Autodesk Inventor part; units mm, degrees
ref_plane "YZ Plane" through (0, 0, 0) normal (1, 0, 0) x (0, 1, 0)
ref_plane "XZ Plane" through (0, 0, 0) normal (0, 1, 0) x (-1, 0, 0)
ref_plane "XY Plane" through (0, 0, 0) normal (0, 0, 1) x (1, 0, 0)
sketch "Sketch2" plane through (0, 0, 0) normal (0, 0, 1) x (1, 0, 0)
  line L0 (0, 0) -> (19, 0)
  line L1 (19, 0) -> (19, 137)
  line L2 (19, 137) -> (0, 137)
  line L3 (0, 137) -> (0, 0)
  dimension "d9" = 19
  dimension "d10" = 137
extrude "Extrusion1" add sketch "Sketch2" along normal blind 19
sketch "Sketch4" plane through (0, 137, 0) normal (0, 1, 0) x (1, 0, 0)
  line L0 (19, 0) -> (0, 0)
  line L1 (0, 0) -> (0, -19)
  line L2 (19, -19) -> (0, -19)
  line L3 (19, 0) -> (19, -19)
  line L4 (1.5, -17.5) -> (1.5, -1.5)
  line L5 (1.5, -1.5) -> (17.5, -1.5)
  line L6 (17.5, -1.5) -> (17.5, -17.5)
  line L7 (17.5, -17.5) -> (1.5, -17.5)
  dimension "d11" = 1.5
extrude "Extrusion3" cut sketch "Sketch4" against normal through all contours L4 L5 L6 L7
properties part number "C009" material "Aluminum 6061"
CAD build for the part. Positions are in the model's coordinates, mm. A direction names the side the tool comes from. Coordinates: 2 decimals unless noted, no trailing zeros. Order: outer loops, then holes, each group sorted by start corner. A loop starts at its lowest first (then second) coordinate and runs counter-clockwise, first axis right, second up. Notation, with made-up numbers: (27, 15.25) -> (69, 15.25) arc R17 ccw to (69, 41.25) -> close; hole circle Ø5 at (87, 49.5). An arc over 180 degrees is marked (long way). Answer in a Markdown table with one row per item.
1) Band-saw the part on A-A (z = 3). List the corners of the cut face in (x, y).
Check values:
| item | result |
|---|---|
| outline | (0, 0) -> (1.5, 0) -> (1.5, 137) -> (0, 137) -> close; (17.5, 0) -> (19, 0) -> (19, 137) -> (17.5, 137) -> close |
2) Drill centre line: line 1 (Z direction, x = 6.75, y = 80). Where is it in solid material? Low to high.
Check values:
| item | result |
|---|---|
| line 1 | 0 to 1.5, 17.5 to 19 |
3) Band-saw the part on B-B (x = 3.75). List the corners of the cut face in (y, z), and give its area (3 significant figures).
Check values:
| item | result |
|---|---|
| outline | (0, 0) -> (137, 0) -> (137, 1.5) -> (0, 1.5) -> close; (0, 17.5) -> (137, 17.5) -> (137, 19) -> (0, 19) -> close |
| area | 411 mm2 |
4) Which spindle directions (+Z, -Z, +X, -X, +Y, -Y) get a long thin tool onto all of the face, cutting with end or side? Do faces 1 (the face through (9, 69, 1.5)), 2 (the face through (18, 137, 9)). Say none if no direction does.
Check values:
| item | result |
|---|---|
| face 1 | +Y, -Y |
| face 2 | +Z, -Z, +X, -X, +Y |
5) Flat gauge pin, fed straight in: P1, Ø10, axis at x = 13.5, z = 14.5, coming from the -Y side. Where does the tip first touch, or does it go through?
Check values:
| item | result |
|---|---|
| P1 | y = 0 |
6) Band-saw the part on C-C (y = 64). List the corners of the cut face in (x, z).
Check values:
| item | result |
|---|---|
| outline | (0, 0) -> (19, 0) -> (19, 19) -> (0, 19) -> close; hole (1.5, 1.5) -> (17.5, 1.5) -> (17.5, 17.5) -> (1.5, 17.5) -> close |
7) Mould opens along X. For faces 3 (the face through (17.5, 69, 9)), 4 (the face through (0, 69, 9)), 5 (the face through (9, 69, 0)) say: pulls with the +X half, pulls with the -X half, needs draft (parallel to the pull), parting line crosses it, or undercut.
Check values:
| item | result |
|---|---|
| face 3 | undercut |
| face 4 | pulls with the -X half |
| face 5 | needs draft |
